Verification items for the finished model (mm, model axes). A direction names the side the tool comes from. Round coordinates to 2 decimals unless told otherwise and drop trailing zeros. Loops run counter-clockwise (first coordinate to the right, second up) from the corner with the lowest first, then second, coordinate; pieces in that order, holes last. Notation, with made-up numbers: M -12.75,89 L 5.25,89 A11 cw 5.25,108 Z; hole C 73,-13 d8. An arc over 180 degrees is marked long. One line per item, written item: value.
Autodesk Inventor part; units mm, degrees
ref_plane "Work Plane11" through (7.5, 24, 70) normal (0, 0, -1) x (-1, 0, 0)
ref_plane "YZ Plane" through (0, 0, 0) normal (1, 0, 0) x (0, 1, 0)
ref_plane "XZ Plane" through (0, 0, 0) normal (0, 1, 0) x (-1, 0, 0)
sketch "Sketch1" plane through (0, 0, 0) normal (0, 1, 0) x (-1, 0, 0)
  arc A0 (-8.9286, 8.7482) -> (8.9286, 8.7482) centre (0, 0) ccw
  line L0 (-7.5, 12.2474) -> (-7.5, 20)
  line L1 (7.5, 20) -> (7.5, 12.2474)
  line L2 (7.5, 20) -> (-7.5, 20)
  arc A1 (7.5, 12.2474) -> (8.9286, 8.7482) centre (12.5, 12.2474) ccw
  arc A2 (-8.9286, 8.7482) -> (-7.5, 12.2474) centre (-12.5, 12.2474) ccw
  point P0 (7.5, 10)
  point P1 (-7.5, 10)
  point P2 (0, 10)
  point P3 (0, 20)
  dimension "d0" = 25
  dimension "d109" = 5
  dimension "d129" = 15
  dimension "d131" = 10
extrude "Extrusion1" add sketch "Sketch1" against normal blind 12
sketch "Sketch22" plane through (-7.5, 0, 20) normal (0, 0, 1) x (1, 0, 0)
  line L0 (0, 0) -> (0, -12)
  line L1 (15, -12) -> (0, -12)
  line L2 (0, 0) -> (15, 0)
  line L3 (15, 0) -> (15, -12)
  line L4 (15, -12) -> (0, -12)
  line L5 (0, -12) -> (0, 0)
  point P0 (7.5, 0)
sketch "Sketch23" plane through (0, 0, 0) normal (1, 0, 0) x (0, 1, 0)
  line L0 (0, 20) -> (-12, 20)
  line L1 (-6, 20) -> (-6, 40)
  line L2 (24, 70) -> (102.7976, 70)
  arc A0 (24, 70) -> (-6, 40) centre (24, 40) ccw
  point P0 (0, 0)
  point P1 (-6, 70)
  dimension "d110" = 50
  dimension "d111" = 108.7976
  dimension "d112" = 90
  dimension "d113" = 30
sweep "Sweep2" add profiles "Sketch22" path "Sketch23" path curves L1 A0 L2
ref_plane "Work Plane11" through (7.5, 24, 70) normal (0, 0, -1) x (-1, 0, 0)
sketch "Sketch24" plane through (7.5, 24, 70) normal (0, 0, -1) x (-1, 0, 0)
  line L0 (0, 78.7976) -> (15, 78.7976)
  line L1 (0, 78.7976) -> (15, 78.7976)
  line L2 (0, 78.7976) -> (0, 82.7508)
  line L3 (15, 78.7976) -> (15, 82.7508)
  arc A0 (15, 82.7508) -> (0, 82.7508) centre (7.5, 90.7976) ccw
  line L4 (0, 78.7976) -> (15, 78.7976)
  point P0 (7.5, -24)
  point P1 (7.5, 78.7976)
  point P2 (7.5, 78.7976)
  dimension "d139" = 22
  dimension "d140" = 12
  dimension "d141" = 15
extrude "Extrusion17" add sketch "Sketch24" along normal mid plane 12
sketch "Sketch25" plane through (-7.5, 24, 76) normal (0, 0, 1) x (1, 0, 0)
  circle A0 centre (7.5, 90.7976) radius 2.5
  arc A1 (15, 82.7508) -> (0, 82.7508) centre (7.5, 90.7976) ccw
  point P0 (7.5, -24)
  dimension "d123" = 5
extrude "Extrusion18" cut sketch "Sketch25" against normal through all
sketch "Sketch27" plane through (0, 0, 0) normal (0, 1, 0) x (1, 0, 0)
  arc A0 (8.9286, -8.7482) -> (-8.9286, -8.7482) centre (0, 0) ccw
  circle A1 centre (0, 0) radius 2.4
  dimension "d136" = 4.8
extrude "Extrusion20" add sketch "Sketch27" against normal blind 26
sketch "Sketch28" plane through (7.5, 24, 64) normal (0, 0, -1) x (-1, 0, 0)
  arc A0 (15, 82.7508) -> (0, 82.7508) centre (7.5, 90.7976) ccw
  circle A1 centre (7.5, 90.7976) radius 8.1
  point P0 (7.5, -24)
  dimension "d142" = 16.2
extrude "Extrusion21" cut sketch "Sketch28" against normal blind 5
mirror "Mirror2" about plane through (7.5, 24, 70) normal (0, 0, -1) of "Extrusion21"
sketch "Sketch29" plane through (0, 0, 0) normal (0, 1, 0) x (1, 0, 0)
  line L0 (3.1754, 0) -> (1.5877, -2.75)
  line L1 (1.5877, -2.75) -> (-1.5877, -2.75)
  line L2 (-1.5877, -2.75) -> (-3.1754, 0)
  line L3 (-3.1754, 0) -> (-1.5877, 2.75)
  line L4 (-1.5877, 2.75) -> (1.5877, 2.75)
  line L5 (1.5877, 2.75) -> (3.1754, 0)
  point P0 (0, 0)
  point P1 (0, 0)
  dimension "d145" = 5.5
extrude "Extrusion22" cut sketch "Sketch29" against normal blind 3
sketch "Sketch30" plane through (0, -3, 0) normal (0, 1, 0) x (1, 0, 0)
  circle A0 centre (0, 0) radius 1.6
  dimension "d148" = 3.2
extrude "Extrusion23" cut sketch "Sketch30" against normal through all
properties part number "distall_link_3"
(1) Depth check by flat-ended pin: pin 1 Ø2 at (x, y) = (4, 19) entering from +Z; pin 2 Ø1.5 at (x, z) = (-8.5, 50.5) entering from -Y; pin 3 Ø8 at (x, y) = (3, 115.5) entering from +Z; pin 4 Ø3.5 at (x, z) = (0, 0) entering from +Y. Enter the tip coordinate at first touch or a pass-through.
Completed:
pin 1: stops at z = 75.78
pin 2: passes through
pin 3: stops at z = 71
pin 4: stops at y = -3
(2) Thickness scan on L1, parallel to X at y = -9, z = 0; L2, parallel to Z at x = 0, y = -16; L3, parallel to Y at x = -4.5, z = 35. Record the ranges inside material, lowest first. Write a range as from..to.
Completed:
L1: x = -12.5..-1.6, 1.6..12.5
L2: z = -2.4..-1.6, 1.6..2.4
L3: y = -12..0
(3) Sectioned sample at B-B on y = -17. Enter the section's corners in (x, z).
Completed:
outline: C 0,0 d4.8; hole C 0,0 d3.2
(4) Mould release check, pull along Y, two halves, no side actions. Record for faces 4 (the face through (7.881, -5.916, 10.333)), 5 (the face through (1.4, -3, -1.3)), 6 (the face through (2, 117, 71)): +Y half, -Y half, draft (parallel to the pull), parting line (faces both ways), or undercut.
Completed:
face 4: draft
face 5: +Y half
face 6: undercut
(5) Sectioned sample at D-D on y = 108.5. Enter the section's corners in (x, z).
Completed:
outline: M -9.02,64 L -5.09,64 L -5.09,69 L 5.09,69 L 5.09,64 L 9.02,64 L 9.02,76 L 5.09,76 L 5.09,71 L -5.09,71 L -5.09,76 L -9.02,76 Z
(6) Tool access check on faces 1 (the face through (-2, 117, 69)), 2 (the face through (0, 64, 64)), 3 (the face through (0, -1, 2.75)). Record the directions out of +Z, -Z, +X, -X, +Y, -Y that give a thin tool (end or side, any length) a straight path to the whole face; none if there is none.
Completed:
face 1: -Z
face 2: -Z, +X, -X, +Y
face 3: +Y
(7) Sectioned sample at A-A on x = 0. Count the separate pieces of the cut face and the enclosed holes in it, and give its area (3 significant figures).
Completed:
separate pieces: 3
enclosed holes: 0
area: 2,220 mm^2
(8) Sectioned sample at C-C on z = 36.5. Enter the section's corners in (x, y).
Completed:
outline: M -7.5,-12 L 7.5,-12 L 7.5,0 L -7.5,0 Z
